Work out the finished part from the listing and answer in its coordinate system (mm). Round coordinates to 2 decimals unless told otherwise and drop trailing zeros. Order: outer loops, then holes, each group sorted by start corner. A loop starts at its lowest first (then second) coordinate and runs counter-clockwise, first axis right, second up. Notation, with made-up numbers: (28, -21) - (83, -21) arc R20 ccw to (83, -9) - close; hole circle Ø5 at (39.5, 77.5). An arc over 180 degrees is marked (long way). Use one line per item in the form item = value. Start each with the question number.
Q1. The part is cut by section B-B on y = 10.5. Determine the outline of the cut face in (x, z), plus the area to 3 significant figures.
Q2. Given P1, Ø2, axis at y = -3.5, z = 9, coming from the +X side; P2, Ø8, axis at y = 30.5, z = 2, coming from the -X side; P3, Ø5, axis at y = -5.5, z = 12.5, coming from the +X side, each flat-ended and moving along its own axis, determine where each tip first touches the part or whether it passes through.
Q3. The part is cut by section C-C on z = -3. Determine the outline of the cut face in (x, y).
Q4. Find the intervals of material crossed by line 1 (Y direction, x = 22.75, z = 26.45); line 2 (Y direction, x = 22, z = -5); line 3 (Z direction, x = 49, y = 3.5), in increasing order. Write a range as [from, to].
Q5. The part is cut by section D-D on x = 30.5. Determine the outline of the cut face in (y, z).
Q6. The part is cut by section A-A on x = 22.75. Determine the outline of the cut face in (y, z).
from build123d import *

# Parameters (mm, degrees)
SKETCH1_R                = 33.358351357
SKETCH1_R_2              = 30.358351357
BOSS_EXTRUDE1_DEPTH      = 25.4
BOSS_EXTRUDE1_DEPTH_BACK = 10
SKETCH2_R                = 33.358351357
SKETCH2_R_2              = 5
BOSS_EXTRUDE2_DEPTH      = 3


with BuildPart() as part:
    # Sketch1 → Boss-Extrude1 (new body, two sides)
    with BuildSketch(Plane.XY) as boss_extrude1_sk:
        with Locations((22.75, 10.5)):
            Circle(SKETCH1_R)
        with Locations((22.75, 10.5)):
            Circle(SKETCH1_R_2, mode=Mode.SUBTRACT)
    extrude(amount=BOSS_EXTRUDE1_DEPTH)
    extrude(boss_extrude1_sk.sketch, amount=-BOSS_EXTRUDE1_DEPTH_BACK)

    # Sketch2 → Boss-Extrude2 (add)
    with BuildSketch(Plane.XY.offset(25.4)):
        with Locations((22.75, 10.5)):
            Circle(SKETCH2_R)
        with Locations((22.75, -8.913617173)):
            Circle(SKETCH2_R_2, mode=Mode.SUBTRACT)
    extrude(amount=BOSS_EXTRUDE2_DEPTH)


solid = part.part
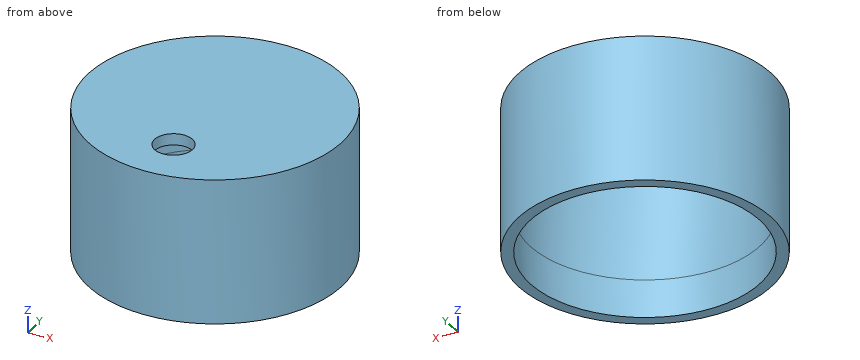
Found:
q1.outline = (-10.61, -10) - (-7.61, -10) - (-7.61, 25.4) - (53.11, 25.4) - (53.11, -10) - (56.11, -10) - (56.11, 28.4) - (-10.61, 28.4) - close
q1.area = 413 mm²
q2.P1 = 53.47
q2.P2 = -6.52
q2.P3 = 53.25
q3.outline = circle Ø66.72 at (22.75, 10.5); hole circle Ø60.72 at (22.75, 10.5)
q4.line_1 = [-22.86, -13.91], [-3.91, 43.86]
q4.line_2 = [-22.85, -19.85], [40.85, 43.85]
q4.line_3 = [25.4, 28.4]
q5.outline = (-21.95, -10) - (-18.85, -10) - (-18.85, 25.4) - (39.85, 25.4) - (39.85, -10) - (42.95, -10) - (42.95, 28.4) - (-21.95, 28.4) - close
q6.outline = (-22.86, -10) - (-19.86, -10) - (-19.86, 25.4) - (-13.91, 25.4) - (-13.91, 28.4) - (-22.86, 28.4) - close; (-3.91, 25.4) - (40.86, 25.4) - (40.86, -10) - (43.86, -10) - (43.86, 28.4) - (-3.91, 28.4) - close
